from build123d import *

# Parameters (mm, degrees)
SKETCH2_R               = 25
SKETCH2_R_2             = 22
EXTRUDE_THIN1_DEPTH     = 60
SKETCH3_W               = 45
SKETCH3_H               = 70
SKETCH3_W_2             = 39
SKETCH3_H_2             = 64
EXTRUDE_THIN2_DEPTH     = 60
SKETCH4_R               = 22
CUT_EXTRUDE1_DEPTH      = 71
CUT_EXTRUDE2_DEPTH      = 26
CUT_EXTRUDE2_DEPTH_BACK = 26
SKETCH6_W               = 39
SKETCH6_H               = 64
CUT_EXTRUDE3_DEPTH      = 50
CUT_EXTRUDE4_DEPTH      = 26
CUT_EXTRUDE4_DEPTH_BACK = 26
SKETCH8_W               = 35
SKETCH8_H               = 39
CUT_EXTRUDE6_DEPTH      = 4
BOSS_EXTRUDE1_DEPTH     = 3
FILLET1_R               = 3
SKETCH10_R              = 6.25
CUT_EXTRUDE7_DEPTH      = 48.5000001
FILLET3_R               = 10
SKETCH11_R              = 12.5
BOSS_EXTRUDE2_DEPTH     = 25


with BuildPart() as part:
    # Sketch2 → Extrude-Thin1 (new body)
    with BuildSketch(Plane(origin=(0, 0, 0), x_dir=(1, 0, 0), z_dir=(0, 1, 0))):
        Circle(SKETCH2_R)
        Circle(SKETCH2_R_2, mode=Mode.SUBTRACT)
    extrude(amount=-EXTRUDE_THIN1_DEPTH)

    # Sketch3 → Extrude-Thin2 (add)
    with BuildSketch(Plane(origin=(0, 0, 0), x_dir=(0, 0, -1), z_dir=(1, 0, 0))):
        with Locations((0, -35)):
            Rectangle(SKETCH3_W, SKETCH3_H)
        with Locations((0, -35)):
            Rectangle(SKETCH3_W_2, SKETCH3_H_2, mode=Mode.SUBTRACT)
    extrude(amount=-EXTRUDE_THIN2_DEPTH)

    # Sketch4 → Cut-Extrude1 (cut, through all)
    with BuildSketch(Plane(origin=(0, 0, 0), x_dir=(1, 0, 0), z_dir=(0, 1, 0))):
        Circle(SKETCH4_R)
    extrude(amount=-CUT_EXTRUDE1_DEPTH, mode=Mode.SUBTRACT)

    # Sketch5 → Cut-Extrude2 (cut, two sides)
    with BuildSketch(Plane.XY) as cut_extrude2_sk:
        Polygon((20, -10), (-50, -90), (25, -90), (25, -10), align=None)
    extrude(amount=CUT_EXTRUDE2_DEPTH, mode=Mode.SUBTRACT)
    extrude(cut_extrude2_sk.sketch, amount=-CUT_EXTRUDE2_DEPTH_BACK, mode=Mode.SUBTRACT)

    # Sketch6 → Cut-Extrude3 (cut)
    with BuildSketch(Plane.ZY.offset(60)):
        with Locations((0, -35)):
            Rectangle(SKETCH6_W, SKETCH6_H)
    extrude(amount=-CUT_EXTRUDE3_DEPTH, mode=Mode.SUBTRACT)

    # Sketch7 → Cut-Extrude4 (cut, two sides)
    with BuildSketch(Plane.XY) as cut_extrude4_sk:
        Polygon((-30, 0), (-60, -70), (-60, 0), align=None)
    extrude(amount=CUT_EXTRUDE4_DEPTH, mode=Mode.SUBTRACT)
    extrude(cut_extrude4_sk.sketch, amount=-CUT_EXTRUDE4_DEPTH_BACK, mode=Mode.SUBTRACT)

    # Sketch8 → Cut-Extrude6 (cut, through all)
    with BuildSketch(Plane(origin=(0, -67, 0), x_dir=(1, 0, 0), z_dir=(0, 1, 0))):
        with Locations((-47.375, 0)):
            Rectangle(SKETCH8_W, SKETCH8_H)
    extrude(amount=-CUT_EXTRUDE6_DEPTH, mode=Mode.SUBTRACT)

    # Sketch9 → Boss-Extrude1 (add)
    with BuildSketch(Plane(origin=(0, 0, 0), x_dir=(1, 0, 0), z_dir=(0, 1, 0))):
        with BuildLine():
            Line((-30, 22.5), (-10.897247359, 22.5))
            ThreePointArc((-10.897247359, 22.5), (25, 0), (-10.897247359, -22.5))
            Line((-10.897247359, -22.5), (-30, -22.5))
            Line((-30, -22.5), (-30, 22.5))
        make_face()
    extrude(amount=-BOSS_EXTRUDE1_DEPTH)

    # Fillet1
    fillet1_edges = [part.edges().sort_by_distance(p)[0] for p in [
        (25, 0, 0),
        (-20.448623679, 0, -22.5),
        (-20.448623679, 0, 22.5),
    ]]
    fillet(fillet1_edges, radius=FILLET1_R)

    # Sketch10 → Cut-Extrude7 (cut, through all)
    with BuildSketch(Plane.XY.offset(22.5)):
        with Locations((-42.5, -60)):
            Circle(SKETCH10_R)
    extrude(amount=-CUT_EXTRUDE7_DEPTH, mode=Mode.SUBTRACT)

    # Fillet3
    fillet3_edges = [part.edges().sort_by_distance(p)[0] for p in [
        (-60, -70, -21),
        (-32.5, -70, -21),
        (-60, -70, 21),
        (-32.5, -70, 21),
    ]]
    fillet(fillet3_edges, radius=FILLET3_R)

    # Sketch11 → Boss-Extrude2 (add)
    with BuildSketch(Plane(origin=(0, 0, 0), x_dir=(1, 0, 0), z_dir=(0, 1, 0))):
        Circle(SKETCH11_R)
    extrude(amount=BOSS_EXTRUDE2_DEPTH)


solid = part.part
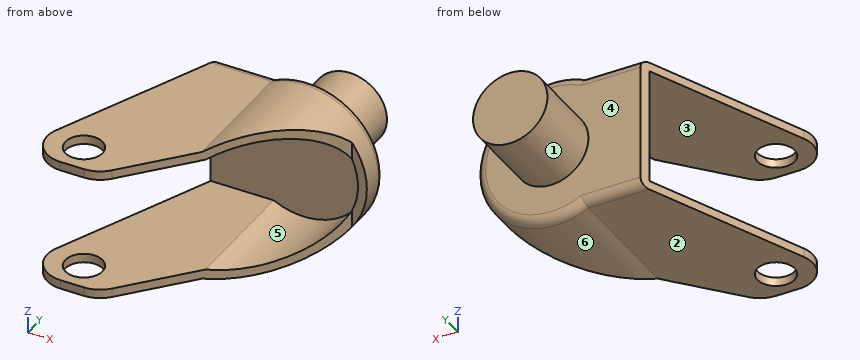
Check sheet for the modelled part. Datum: model origin and axes. Units: mm. Face numbers are marked on the shaded views. A direction names the side the tool comes from. Round coordinates to 2 decimals unless told otherwise and drop trailing zeros. Loops run counter-clockwise (first coordinate to the right, second up) from the corner with the lowest first, then second, coordinate; pieces in that order, holes last. Notation, with made-up numbers: (13.25, -8.75) - (68.25, -8.75) arc R21 ccw to (68.25, 23.25) - close; hole circle Ø9 at (66.25, -27.75). An arc over 180 degrees is marked (long way). Answer as CSV lines item,"result". Start each with the question number.
Item 1: Section check B-B (z = 0). Record the boundary of the cut face in (x, y).
Item 2: Scan lines: line 1 (Z direction, x = -21, y = -30.5); line 2 (Z direction, x = 0, y = -15.5); line 3 (Y direction, x = 4.5, z = -9). Record each from-to range of solid material in increasing order. Write a range as [from, to].
Item 3: Depth check by flat-ended pin: P1, Ø1.5, axis at x = -35.5, y = -33, coming from the +Z side; P2, Ø22, axis at x = -2, z = -2.5, coming from the -Y side; P3, Ø2.5, axis at x = 22.5, z = 6, coming from the -Y side. Enter the tip coordinate at first touch or a pass-through.
Item 4: Section check A-A (y = -60). Record the boundary of the cut face in (x, z), and give its area (3 significant figures).
Item 5: Release check for a two-part mould opening along Z. For the marked faces 4, 5 and 6 record: +Z half, -Z half, draft (parallel to the pull), parting line (faces both ways), or undercut.
Item 6: Section check C-C (y = -25.5). Record the boundary of the cut face in (x, z).
Item 7: Set-up check for the marked faces 1, 2 and 3: record each of +Z, -Z, +X, -X, +Y, -Y from which the full face is reachable in a straight line by a thin tool's end or side.
Item 8: Section check D-D (x = 0). Record the boundary of the cut face in (y, z), and give its area (3 significant figures).
Report:
1,outline,"(-31.29, -3) - (22, -3) - (22, -10) - (25, -10) - (25, -3) arc R3 ccw to (22, 0) - (12.5, 0) - (12.5, 25) - (-12.5, 25) - (-12.5, 0) - (-30, 0) - close"
2,line 1,"z = [-22.5, -19.5], [19.5, 22.5]"
2,line 2,"z = [-25, -22], [22, 25]"
2,line 3,"y = [-3, 25]"
3,P1,"stops at z = 22.5"
3,P2,"stops at y = -3"
3,P3,"stops at y = -10"
4,outline,"(-54.83, -22.5) - (-48.75, -22.5) - (-48.75, -19.5) - (-54.83, -19.5) - close; (-54.83, 19.5) - (-48.75, 19.5) - (-48.75, 22.5) - (-54.83, 22.5) - close; (-36.25, -22.5) - (-23.75, -22.5) - (-23.75, -19.5) - (-36.25, -19.5) - close; (-36.25, 19.5) - (-23.75, 19.5) - (-23.75, 22.5) - (-36.25, 22.5) - close"
4,area,"112 mm2"
5,face 4,"draft"
5,face 5,"undercut"
5,face 6,"parting line"
6,outline,"(-40.93, -22.5) - (-10.9, -22.5) arc R25 ccw to (6.44, -24.16) - (6.44, -21.04) arc R22 cw to (-10.19, -19.5) - (-40.93, -19.5) - close; (-40.93, 19.5) - (-10.19, 19.5) arc R22 cw to (6.44, 21.04) - (6.44, 24.16) arc R25 ccw to (-10.9, 22.5) - (-40.93, 22.5) - close"
7,face 1,"+Y"
7,face 2,"-Z, -X, +Y, -Y"
7,face 3,"-X, -Y"
8,outline,"(-32.86, -25) - (-3, -25) arc R3 ccw to (0, -22) - (0, -12.5) - (25, -12.5) - (25, 12.5) - (0, 12.5) - (0, 22) arc R3 ccw to (-3, 25) - (-32.86, 25) - (-32.86, 22) - (-3, 22) - (-3, -22) - (-32.86, -22) - close"
8,area,"950 mm2"
